from build123d import *

# Parameters (mm, degrees)
BOSS_EXTRUDE1_DEPTH               = 507
TAP_DRILL_FOR_M5_TAP1_D           = 5.2
TAP_DRILL_FOR_M5_TAP1_DEPTH       = 46
TAP_DRILL_FOR_M5_TAP1_CSINK_D     = 6
TAP_DRILL_FOR_M5_TAP1_CSINK_ANGLE = 90
TAP_DRILL_FOR_M5_TAP1_TIP         = 1.562237609


with BuildPart() as part:
    # Sketch1 → Boss-Extrude1 (new body)
    with BuildSketch(Plane.XY):
        Polygon((5.5, 3), (-5.5, 3), (-5.5, 0), (-22.5, 0), (-22.5, 5), (-9.597702448, 5), (-3.67559519, 17.7), (0, 15.986041815), (3.67559519, 17.7), (9.597702448, 5), (22.5, 5), (22.5, 0), (5.5, 0), align=None)
    extrude(amount=BOSS_EXTRUDE1_DEPTH)

    # Tap Drill for M5 Tap1
    with Locations(Plane(origin=(-15, 5, 12), x_dir=(0, 0, 1), z_dir=(0, 1, 0))):
        with Locations((0, 0), (0, 30), (80, 0), (80, 30), (180, 0), (180, 30), (280, 0), (280, 30), (380, 0), (380, 30), (480, 0), (480, 30)):
            CounterSinkHole(TAP_DRILL_FOR_M5_TAP1_D / 2, TAP_DRILL_FOR_M5_TAP1_CSINK_D / 2, depth=TAP_DRILL_FOR_M5_TAP1_DEPTH, counter_sink_angle=TAP_DRILL_FOR_M5_TAP1_CSINK_ANGLE)
            with Locations((0, 0, -(TAP_DRILL_FOR_M5_TAP1_DEPTH + TAP_DRILL_FOR_M5_TAP1_TIP / 2))):  # 118° drill point
                Cone(0, TAP_DRILL_FOR_M5_TAP1_D / 2, TAP_DRILL_FOR_M5_TAP1_TIP, mode=Mode.SUBTRACT)


solid = part.part
The listing builds one solid part. Answer for the finished solid, in the listing's coordinates (mm). A direction names the side the tool comes from. Give positions to 0.01 mm unless a question says otherwise; leave off trailing zeros. Order: outer loops, then holes, each group sorted by start corner. A loop starts at its lowest first (then second) coordinate and runs counter-clockwise, first axis right, second up. Notation, with made-up numbers: (-26.75, 0) - (14.25, 0) arc R16 cw to (14.25, 27) - close; hole circle Ø1 at (43, 32). An arc over 180 degrees is marked (long way). One line per item, written item: value. Start each with the question number.
1) A cutting plane is placed at B-B on y = 13.25. Give the vertices of the cut face in (x, z), then the cut area to 3 significant figures.
2) A cutting plane is placed at A-A on z = 257. Give the vertices of the cut face in (x, y).
3) Find the intervals of material crossed by L1, parallel to X at y = 1, z = 192; L2, parallel to Y at x = 16.5, z = 471.5; L3, parallel to X at y = 2, z = 402, in increasing order.
4) A tool of negligible diameter and unlimited length cuts with its end or side. For faces 1 (the face through (16, 5, 250)), 2 (the face through (-14, 0, 250)), from which of +Z, -Z, +X, -X, +Y, -Y can it reach the whole face along a straight path? Write none if from no direction.
5) Given pin 1 Ø14 at (x, z) = (15.5, 256) entering from +Y; pin 2 Ø3 at (x, z) = (-15, 192) entering from -Y; pin 3 Ø6 at (y, z) = (15, 323.5) entering from +X; pin 4 Ø4 at (y, z) = (9, 341.5) entering from +X, each flat-ended and moving along its own axis, determine where each tip first touches the part or whether it passes through.
6) The mould has two halves that part along X. Classify faces 3 (the face through (-16, 5, 250)), 4 (the face through (-6.68, 11.26, 249.95)), 5 (the face through (6.595, 11.439, 249.951)), 6 (the face through (0, 3, 250)): released by +X, released by -X, zero draft, split by the parting line, or undercut.
Answer sheet:
1. outline: (-5.75, 0) - (5.75, 0) - (5.75, 507) - (-5.75, 507) - close
1. area: 5,830 mm2
2. outline: (-22.5, 0) - (-5.5, 0) - (-5.5, 3) - (5.5, 3) - (5.5, 0) - (22.5, 0) - (22.5, 5) - (9.6, 5) - (3.68, 17.7) - (0, 15.99) - (-3.68, 17.7) - (-9.6, 5) - (-22.5, 5) - close
3. L1: x = -22.5 to -17.6, -12.4 to -5.5, 5.5 to 12.4, 17.6 to 22.5
3. L2: y = 0 to 5
3. L3: x = -22.5 to -5.5, 5.5 to 22.5
4. face 1: +Z, -Z, +X, +Y
4. face 2: +Z, -Z, +X, -X, -Y
5. pin 1: stops at y = 7.35
5. pin 2: passes through
5. pin 3: stops at x = 6.33
5. pin 4: stops at x = 8.67
6. face 3: zero draft
6. face 4: released by -X
6. face 5: released by +X
6. face 6: undercut
